from build123d import *

# Parameters (mm, degrees)
BOSS_EXTRUDE1_DEPTH   = 6
SHELL1_T              = -2
SKETCH2_R             = 2.75
BOSS_EXTRUDE2_DEPTH   = 3
SKETCH2_R_2           = 4.5
BOSS_EXTRUDE2_2_DEPTH = 3
BOSS_EXTRUDE2_3_DEPTH = 3
BOSS_EXTRUDE3_START   = 5
SKETCH3_R             = 4.5
SKETCH3_R_2           = 4.25
BOSS_EXTRUDE3_DEPTH   = 5
SKETCH4_R             = 3.25
CUT_EXTRUDE1_DEPTH    = 2
SKETCH5_R             = 1.75
CUT_EXTRUDE2_DEPTH    = 73.907475611
BOSS_EXTRUDE5_START   = 2
SKETCH7_R             = 11
BOSS_EXTRUDE5_DEPTH   = 2
SKETCH6_R             = 1.25
SKETCH6_R_2           = 6
CUT_EXTRUDE4_DEPTH    = 73.687688091
SKETCH9_R             = 10
BOSS_EXTRUDE6_DEPTH   = 4


with BuildPart() as part:
    # Sketch1 → Boss-Extrude1 (new body)
    with BuildSketch(Plane(origin=(0, 0, 0), x_dir=(1, 0, 0), z_dir=(0, 1, 0))):
        with BuildLine():
            Line((-17.502255184, 15.174365801), (-26.545454545, 11.644262234))
            ThreePointArc((-26.545454545, 11.644262234), (-34.5, 0), (-26.545454545, -11.644262234))
            Line((-26.545454545, -11.644262234), (-17.502255184, -15.174365801))
            ThreePointArc((-17.502255184, -15.174365801), (-12.363636364, -13.808065596), (-9.50963812, -18.294364031))
            Line((-9.50963812, -18.294364031), (11.636363636, -26.548917894))
            ThreePointArc((11.636363636, -26.548917894), (50.5, 0), (11.636363636, 26.548917894))
            Line((11.636363636, 26.548917894), (-9.50963812, 18.294364031))
            ThreePointArc((-9.50963812, 18.294364031), (-12.363636364, 13.808065596), (-17.502255184, 15.174365801))
        make_face()
    extrude(amount=BOSS_EXTRUDE1_DEPTH)

    # Shell1
    shell1_openings = [part.faces().sort_by_distance(p)[0] for p in [
        (12.478104295, 6, 0),
    ]]
    offset(amount=SHELL1_T, openings=shell1_openings, kind=Kind.INTERSECTION)



with BuildPart() as body_2:
    # Sketch2 → Boss-Extrude2 (new body)
    with BuildSketch(Plane.XZ):
        with BuildLine():
            Line((49.626979567, -7), (63.125355805, -4.158876316))
            ThreePointArc((63.125355805, -4.158876316), (66.5, 0), (63.125355805, 4.158876316))
            Line((63.125355805, 4.158876316), (49.626979567, 7))
            ThreePointArc((49.626979567, 7), (50.5, 0), (49.626979567, -7))
        make_face()
        with Locations(Location((62.25, 0, 0), (0, 0, 270))):
            Circle(SKETCH2_R, mode=Mode.SUBTRACT)
    extrude(amount=-BOSS_EXTRUDE2_DEPTH)


with BuildPart() as body_3:
    # Sketch2 → Boss-Extrude2 2 (new body)
    with BuildSketch(Plane.XZ):
        with Locations(Location((-14, -18, 0), (0, 0, 270))):
            Circle(SKETCH2_R_2)
        with Locations(Location((-14, -18, 0), (0, 0, 270))):
            Circle(SKETCH2_R, mode=Mode.SUBTRACT)
    extrude(amount=-BOSS_EXTRUDE2_2_DEPTH)


with BuildPart() as body_4:
    # Sketch2 → Boss-Extrude2 3 (new body)
    with BuildSketch(Plane.XZ):
        with Locations(Location((-14, 18, 0), (0, 0, 90))):
            Circle(SKETCH2_R_2)
        with Locations(Location((-14, 18, 0), (0, 0, 90))):
            Circle(SKETCH2_R, mode=Mode.SUBTRACT)
    extrude(amount=-BOSS_EXTRUDE2_3_DEPTH)


with BuildPart() as part_1:
    add(part.part)

    add(body_2.part)  # Boss-Extrude3 merges body 2

    add(body_3.part)  # Boss-Extrude3 merges body 3

    add(body_4.part)  # Boss-Extrude3 merges body 4
    # Sketch3 → Boss-Extrude3 (add)
    with BuildSketch(Plane.XZ.offset(BOSS_EXTRUDE3_START)):
        with Locations(Location((-14, 18, 0), (0, 0, 270))):
            Circle(SKETCH3_R)
        with Locations(Location((62.25, 0, 0), (0, 0, 270))):
            Circle(SKETCH3_R_2)
        with Locations(Location((-14, -18, 0), (0, 0, 270))):
            Circle(SKETCH3_R)
    extrude(amount=-BOSS_EXTRUDE3_DEPTH)

    # Sketch4 → Cut-Extrude1 (cut)
    with BuildSketch(Plane.XZ.offset(5)):
        with Locations(Location((-14, 18, 0), (0, 0, 270))):
            Circle(SKETCH4_R)
        with Locations(Location((-14, -18, 0), (0, 0, 90))):
            Circle(SKETCH4_R)
        with Locations(Location((62.25, 0, 0), (0, 0, 270))):
            Circle(SKETCH4_R)
    extrude(amount=-CUT_EXTRUDE1_DEPTH, mode=Mode.SUBTRACT)

    # Sketch5 → Cut-Extrude2 (cut, through all)
    with BuildSketch(Plane.XZ.offset(3)):
        with Locations(Location((-14, 18, 0), (0, 0, 270))):
            Circle(SKETCH5_R)
        with Locations(Location((-14, -18, 0), (0, 0, 270))):
            Circle(SKETCH5_R)
        with Locations(Location((62.25, 0, 0), (0, 0, 270))):
            Circle(SKETCH5_R)
    extrude(amount=-CUT_EXTRUDE2_DEPTH, mode=Mode.SUBTRACT)

    # Sketch7 → Boss-Extrude5 (add)
    with BuildSketch(Plane.XZ.offset(BOSS_EXTRUDE5_START)):
        with Locations(Location((-22, 0, 0), (0, 0, 90))):
            Circle(SKETCH7_R)
        with BuildLine():
            ThreePointArc((48.5, 0), (30.585718173, 25.070609156), (1.063362758, 16.245221482))
            Line((1.063362758, 16.245221482), (1.063362758, -16.245221482))
            ThreePointArc((1.063362758, -16.245221482), (30.585718173, -25.070609156), (48.5, 0))
        make_face()
    extrude(amount=-BOSS_EXTRUDE5_DEPTH)

    # Sketch6 → Cut-Extrude4 (cut, through all)
    with BuildSketch(Plane(origin=(0, 2, 0), x_dir=(1, 0, 0), z_dir=(0, 1, 0))):
        with Locations(Location((-29.5, 0, 0), (0, 0, 270))):
            Circle(SKETCH6_R)
        with Locations(Location((-18.25, 6.495190528, 0), (0, 0, 270))):
            Circle(SKETCH6_R)
        with Locations(Location((-18.25, -6.495190528, 0), (0, 0, 270))):
            Circle(SKETCH6_R)
        with Locations(Location((-22, 0, 0), (0, 0, 270))):
            Circle(SKETCH6_R_2)
    extrude(amount=-CUT_EXTRUDE4_DEPTH, mode=Mode.SUBTRACT)

    # Sketch9 → Boss-Extrude6 (add)
    with BuildSketch(Plane(origin=(0, 2, 0), x_dir=(1, 0, 0), z_dir=(0, 1, 0))):
        with Locations(Location((22, 0, 0), (0, 0, 270))):
            Circle(SKETCH9_R)
    extrude(amount=BOSS_EXTRUDE6_DEPTH)


solid = part_1.part
Can you work these out from the model? Positions are in its coordinate system, mm. A direction names the side the tool comes from. Coordinates: 2 decimals unless noted, no trailing zeros. Loops run counter-clockwise (first coordinate to the right, second up) from the corner with the lowest first, then second, coordinate; pieces in that order, holes last. Notation, with made-up numbers: (-12, 25.25) - (22, 25.25) arc R14 cw to (22, 41.25) - close; hole circle Ø6 at (-24.75, 88). An arc over 180 degrees is marked (long way). Answer as a JSON object with one key per item and string values. Group by question number.
Item 1: If we mould it in two halves opening along X, with no side actions, what happens to faces 1 (the face through (-28.446, 0.028, 0.672)), 2 (the face through (-11, 3, 18)), 3 (the face through (-21.961, 2.958, -13.434)), 4 (the face through (56.28, 1.48, -5.6))? For each: released by +X, released by -X, zero draft, split by the parting line, or undercut.
Item 2: On a 3-axis mill with a long thin cutter (end or side, diameter ignored), from which of +Z, -Z, +X, -X, +Y, -Y can I reach the whole of each face in a straight line? I mean faces 5 (the face through (-12.141, 1.479, -15.973)), 6 (the face through (0.915, 2.958, 22.364)), 7 (the face through (-17, 3, -18)), 8 (the face through (-12.6, -3, -16.6)). Say none if no direction works.
Item 3: If we section it at D-D (x = 37): List the corners of the cut face in (y, z) for me, plus the area to 3 significant figures.
Item 4: For pin 1 (5 mm diameter, centred on x = -14, z = 18, fed in from +Y); pin 2 (4 mm diameter, centred on x = -15.5, y = -2.5, fed in from -Z); pin 3 (6 mm diameter, centred on y = 3.5, z = 13, fed in from +X); pin 4 (7 mm diameter, centred on x = -22, z = 0, fed in from -Y), each with a flat end and sliding along its axis, tell me the tip position at first contact or that it passes through.
Item 5: If we section it at A-A (y = 4.25): List the corners of the cut face in (x, z) for me.
Item 6: If I drill on L1, parallel to X at y = -0.2, z = 0; L2, parallel to X at y = 4, z = -8.5; L3, parallel to Z at x = 14.5, y = 4.75, over which ranges is the centre line in solid material (lowest first)? Write a range as from..to.
Item 7: If we section it at C-C (x = -22): List the corners of the cut face in (y, z) for me.
Item 8: If we section it at B-B (x = 22): List the corners of the cut face in (y, z) for me, plus the area to 3 significant figures.
Returned:
{
 "1": {"face 1": "undercut", "face 2": "undercut", "face 3": "released by -X", "face 4": "released by +X"},
 "2": {"face 5": "+Y", "face 6": "+Z, +Y, -Y", "face 7": "-Z, +Y", "face 8": "-Y"},
 "3": {"outline": "(-2, -21.85) - (0, -21.85) - (0, -24.23) - (6, -24.23) - (6, -21.85) - (2, -21.85) - (2, 21.85) - (6, 21.85) - (6, 24.23) - (0, 24.23) - (0, 21.85) - (-2, 21.85) - close", "area": "203 mm²"},
 "4": {"pin 1": "stops at y = 0", "pin 2": "stops at z = -22.5", "pin 3": "stops at x = 48.69", "pin 4": "passes through"},
 "5": {"outline": "(-26.55, -11.64) - (-17.5, -15.17) arc R4.5 cw to (-9.51, -18.29) - (11.64, -26.55) arc R28.5 ccw (long way) to (11.64, 26.55) - (-9.51, 18.29) arc R4.5 cw to (-17.5, 15.17) - (-26.55, 11.64) arc R12.5 ccw to start; circle Ø20 at (22, 0); hole (-25.82, -9.78) - (-17.96, -12.85) arc R6.5 cw to (-7.59, -16.89) - (12.36, -24.69) arc R26.5 ccw (long way) to (12.36, 24.69) - (-7.59, 16.89) arc R6.5 cw to (-17.96, 12.85) - (-25.82, 9.78) arc R10.5 ccw to start"},
 "6": {"L1": "x = -33..-30.75, -28.25..-28, -16..-11, 1.06..48.5, 58..60.5, 64..66.5", "L2": "x = -31.17..-28.16, 16.73..27.27, 47.1..49.2", "L3": "z = -27.5..-25.42, -6.61..6.61, 25.42..27.5"},
 "7": {"outline": "(-2, -11) - (0, -11) - (0, -13.42) - (6, -13.42) - (6, -11.27) - (2, -11.27) - (2, -6) - (-2, -6) - close; (-2, 6) - (2, 6) - (2, 11.27) - (6, 11.27) - (6, 13.42) - (0, 13.42) - (0, 11) - (-2, 11) - close"},
 "8": {"outline": "(-2, -26.5) - (0, -26.5) - (0, -28.5) - (6, -28.5) - (6, -26.5) - (2, -26.5) - (2, -10) - (6, -10) - (6, 10) - (2, 10) - (2, 26.5) - (6, 26.5) - (6, 28.5) - (0, 28.5) - (0, 26.5) - (-2, 26.5) - close", "area": "316 mm²"}
}
